Here's how the part is built. I have some questions about the finished solid (model axes, mm). Face numbers are marked on the shaded views. A direction names the side the tool comes from. Coordinates: 2 decimals unless noted, no trailing zeros. Loops run counter-clockwise (first coordinate to the right, second up) from the corner with the lowest first, then second, coordinate; pieces in that order, holes last. Notation, with made-up numbers: M 55.5,-19 L 90.5,-19 A29 ccw 90.5,10 Z; hole C 30.5,41 d9. An arc over 180 degrees is marked long. Use CSV: the item, a comma, the result in double quotes. Start each with the question number.
Q1. Please list where these lines run through material, in increasing order: probe 1 along X at (y, z) = (20.5, -35.5) (3 decimals); probe 2 along Y at (x, z) = (28, 26) (3 decimals). Write a range as [from, to].
Q2. If we section it at B-B (x = -29): Please give me the cut outline in (y, z) (3 decimals).
Q3. If we section it at A-A (y = -16.5): Please give me the cut outline in (x, z) (3 decimals).
Q4. If we mould it in two halves opening along Y, with no side actions, what happens to the marked faces 1, 2 and 3? For each: +Y half, -Y half, draft (parallel to the pull), parting line (faces both ways), or undercut.
Q5. If we section it at C-C (z = 40): Please give me the cut outline in (x, y) (3 decimals), and give its area (3 significant figures).
Q6. Which directions (+Z, -Z, +X, -X, +Y, -Y) give clear straight access to the entire face, cutting with the end or side of a thin tool? Please do the marked faces 4 and 5.
Autodesk Inventor part; units mm, degrees
ref_plane "YZ Plane" through (0, 0, 0) normal (1, 0, 0) x (0, 1, 0)
ref_plane "XZ Plane" through (0, 0, 0) normal (0, 1, 0) x (-1, 0, 0)
ref_plane "XY Plane" through (0, 0, 0) normal (0, 0, 1) x (1, 0, 0)
sketch "Sketch1" plane through (0, 0, 0) normal (0, 0, 1) x (1, 0, 0)
  line L0 (-71.12, 0) -> (71.12, 0) construction
  line L1 (0, -35.56) -> (0, 35.56) construction
  line L2 (-50.8, 25.4) -> (50.8, 25.4)
  line L3 (50.8, 25.4) -> (50.8, -25.4)
  line L4 (50.8, -25.4) -> (-50.8, -25.4)
  line L5 (-50.8, -25.4) -> (-50.8, 25.4)
  line L6 (-47.625, 22.225) -> (47.625, 22.225)
  line L7 (47.625, 22.225) -> (47.625, -22.225)
  line L8 (47.625, -22.225) -> (-47.625, -22.225)
  line L9 (-47.625, -22.225) -> (-47.625, 22.225)
  point P0 (0, 0)
  point P1 (-50.8, 0)
  point P2 (0, 25.4)
  point P3 (-47.625, 0)
  point P4 (0, 22.225)
  dimension "d0" = 50.8
  dimension "d1" = 3.175
  dimension "d11" = 101.6
  dimension "d12" = 3.175
extrude "Extrusion1" add sketch "Sketch1" along normal mid plane 101.6
equation "\"d12\" = d1"
properties part number "Arm 4 inch" material "Aluminum 6061"
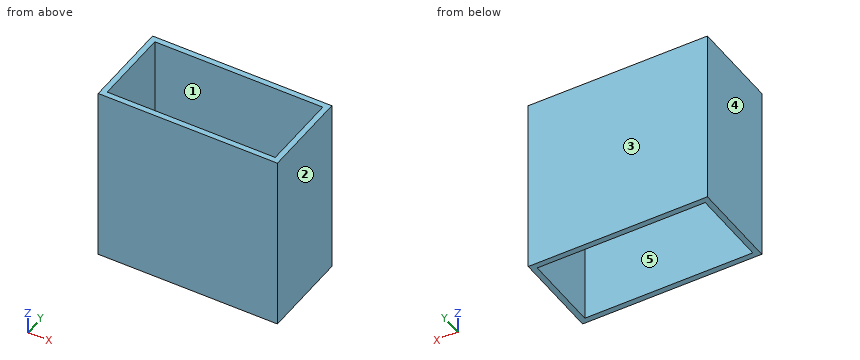
Results below:
1,probe 1,"[-50.8, -47.625], [47.625, 50.8]"
1,probe 2,"[-25.4, -22.225], [22.225, 25.4]"
2,outline,"M -25.4,-50.8 L -22.225,-50.8 L -22.225,50.8 L -25.4,50.8 Z; M 22.225,-50.8 L 25.4,-50.8 L 25.4,50.8 L 22.225,50.8 Z"
3,outline,"M -50.8,-50.8 L -47.625,-50.8 L -47.625,50.8 L -50.8,50.8 Z; M 47.625,-50.8 L 50.8,-50.8 L 50.8,50.8 L 47.625,50.8 Z"
4,face 1,"undercut"
4,face 2,"draft"
4,face 3,"+Y half"
5,outline,"M -50.8,-25.4 L 50.8,-25.4 L 50.8,25.4 L -50.8,25.4 Z; hole M -47.625,-22.225 L 47.625,-22.225 L 47.625,22.225 L -47.625,22.225 Z"
5,area,"927 mm^2"
6,face 4,"+Z, -Z, -X, +Y, -Y"
6,face 5,"+Z, -Z"
